from build123d import *

# Parameters (mm, degrees)
SKETCH1_W           = 10
SKETCH1_H           = 5
BOSS_EXTRUDE1_DEPTH = 3
CUT_EXTRUDE9_DEPTH  = 12.874342087
SKETCH20_R          = 1.5
CUT_EXTRUDE11_DEPTH = 1.2
CUT_EXTRUDE12_START = -0.3
SKETCH22_R          = 1.5
SKETCH22_R_2        = 0.55
CUT_EXTRUDE12_DEPTH = 0.3
SKETCH24_W          = 0.8
SKETCH24_H          = 0.6
CUT_EXTRUDE13_DEPTH = 12.874342087


with BuildPart() as part:
    # Sketch1 → Boss-Extrude1 (new body)
    with BuildSketch(Plane(origin=(0, 4, 0), x_dir=(-1, 0, 0), z_dir=(0, 1, 0))):
        with Locations((-5, 2.5)):
            Rectangle(SKETCH1_W, SKETCH1_H)
    extrude(amount=-BOSS_EXTRUDE1_DEPTH)

    # Sketch18 → Cut-Extrude9 (cut, through all)
    with BuildSketch(Plane(origin=(10, 0, 0), x_dir=(0, 0, -1), z_dir=(1, 0, 0))):
        Polygon((-3.4, 3.4), (-4, 2.360769515), (-3.4, 2.360769515), (-3.4, 2.110769515), (-1.6, 2.110769515), (-1.6, 2.360769515), (-1, 2.360769515), (-1.6, 3.4), (-1.6, 4), (-3.4, 4), align=None)
    extrude(amount=-CUT_EXTRUDE9_DEPTH, mode=Mode.SUBTRACT)

    # Sketch20 → Cut-Extrude11 (cut)
    with BuildSketch(Plane.ZY):
        with Locations((2.5, 3.060769515)):
            Circle(SKETCH20_R)
    extrude(amount=-CUT_EXTRUDE11_DEPTH, mode=Mode.SUBTRACT)

    # Sketch22 → Cut-Extrude12 (cut)
    with BuildSketch(Plane(origin=(10, 0, 0), x_dir=(0, 0, -1), z_dir=(1, 0, 0)).offset(CUT_EXTRUDE12_START)):
        with Locations((-2.5, 3.060769515)):
            Circle(SKETCH22_R)
        with Locations((-2.5, 3.060769515)):
            Circle(SKETCH22_R_2, mode=Mode.SUBTRACT)
    extrude(amount=CUT_EXTRUDE12_DEPTH, mode=Mode.SUBTRACT)

    # Sketch24 → Cut-Extrude13 (cut, through all)
    with BuildSketch(Plane.XY.offset(5)):
        with Locations((2.2, 1.3)):
            Rectangle(SKETCH24_W, SKETCH24_H)
    extrude(amount=-CUT_EXTRUDE13_DEPTH, mode=Mode.SUBTRACT)


solid = part.part
Work out the finished part from the listing and answer in its coordinate system (mm). A direction names the side the tool comes from. Give positions to 0.01 mm unless a question says otherwise; leave off trailing zeros. Loops run counter-clockwise (first coordinate to the right, second up) from the corner with the lowest first, then second, coordinate; pieces in that order, holes last. Notation, with made-up numbers: (-1, 14) -> (21, 14) arc R29 ccw to (21, 51) -> close; hole circle Ø3 at (15, 8.5). An arc over 180 degrees is marked (long way). Use a Markdown table: item, result. Add a question column.
1) The part is cut by section A-A, the plane z = 2.5. Determine the outline of the cut face in (x, y).
2) Which of the six approach directions +Z, -Z, +X, -X, +Y, -Y give full straight-line access (tool end or side, diameter ignored) to faces 4 (the cylindrical face through (0.59, 1.56, 2.48)), 5 (the cylindrical face through (9.85, 1.56, 2.52)), 6 (the flat face through (5, 3, 5))?
3) For a pull along Y with two mould halves and no side action, classify faces 1 (the flat face through (6, 2.111, 3)), 2 (the flat face through (5.07, 2.888, 3.696)), 3 (the flat face through (2, 1.6, 3)) as +Y half, -Y half, draft (parallel to the pull), parting line (faces both ways), or undercut.
4) The part is cut by section C-C, the plane y = 2.95. Determine the outline of the cut face in (x, z), plus the area to 3 significant figures.
5) This flat-tipped pin is pushed along its axis until it touches: P1, Ø0.7, axis at y = 3.5, z = 1.5, coming from the +X side. Where does it stop, or does it pass through?
6) The part is cut by section B-B, the plane x = 8. Determine the outline of the cut face in (y, z).
7) Consider line 1 along X through (y, z) = (1.35, 0.35); line 2 along Z through (x, y) = (5.5, 3.75); line 3 along Y through (x, z) = (5.25, 1.7). Determine where each line is inside the solid, lowest interval first.
8) The part is cut by section D-D, the plane z = 1.5. Determine the outline of the cut face in (x, y).
Reported:
| question | item | result |
|---|---|---|
| 1 | outline | (0, 1) -> (1.8, 1) -> (1.8, 1.6) -> (2.6, 1.6) -> (2.6, 1) -> (10, 1) -> (10, 1.56) -> (9.7, 1.56) -> (9.7, 2.11) -> (1.2, 2.11) -> (1.2, 1.56) -> (0, 1.56) -> close |
| 2 | face 4 | -X |
| 2 | face 5 | +X |
| 2 | face 6 | +Z, +X, -X, +Y, -Y |
| 3 | face 1 | +Y half |
| 3 | face 2 | undercut |
| 3 | face 3 | -Y half |
| 4 | outline | (0, 0) -> (10, 0) -> (10, 1) -> (9.7, 1) -> (9.7, 1.34) -> (1.2, 1.34) -> (1.2, 1) -> (0, 1) -> close; (0, 4) -> (1.2, 4) -> (1.2, 3.66) -> (9.7, 3.66) -> (9.7, 4) -> (10, 4) -> (10, 5) -> (0, 5) -> close |
| 4 | area | 25.8 mm^2 |
| 5 | P1 | stops at x = 9.7 |
| 6 | outline | (1, 0) -> (4, 0) -> (4, 1.6) -> (3.4, 1.6) -> (2.36, 1) -> (2.36, 1.6) -> (2.11, 1.6) -> (2.11, 3.4) -> (2.36, 3.4) -> (2.36, 4) -> (3.4, 3.4) -> (4, 3.4) -> (4, 5) -> (1, 5) -> close |
| 7 | line 1 | x = 0 to 1.8, 2.6 to 10 |
| 7 | line 2 | z = 0 to 1.6, 3.4 to 5 |
| 7 | line 3 | y = 1 to 2.11 |
| 8 | outline | (0, 1) -> (1.8, 1) -> (1.8, 1.6) -> (2.6, 1.6) -> (2.6, 1) -> (10, 1) -> (10, 1.94) -> (9.7, 1.94) -> (9.7, 2.36) -> (1.2, 2.36) -> (1.2, 1.94) -> (0, 1.94) -> close; (1.2, 3.23) -> (9.7, 3.23) -> (9.7, 4) -> (1.2, 4) -> close |
